```python
from build123d import *

# Parameters (mm, degrees)
SKETCH1_W                                  = 90
SKETCH1_H                                  = 65
SKETCH1_R                                  = 1.1
BOSS_EXTRUDE1_DEPTH                        = 1.6
CELL_AND_THERMISTOR_CONNECTORS_OUTLINE_W   = 29.4
CELL_AND_THERMISTOR_CONNECTORS_OUTLINE_H   = 11.5
CELL_AND_THERMISTOR_CONNECTORS_OUTLINE_W_2 = 27.4
CELL_AND_THERMISTOR_CONNECTORS_OUTLINE_H_2 = 9.5
CELL_AND_THERMISTOR_CONNECTORS_OUTLINE_W_3 = 11.4
CELL_AND_THERMISTOR_CONNECTORS_OUTLINE_W_4 = 9.4
CELL_AND_THERMISTOR_CONNECTORS_DEPTH       = 9.25
SKETCH3_W                                  = 13.5
SKETCH3_H                                  = 19.5
BOSS_EXTRUDE2_DEPTH                        = 19.5
SKETCH4_R                                  = 6
BOSS_EXTRUDE3_DEPTH                        = 13.5
SKETCH5_W                                  = 4.83
SKETCH5_H                                  = 17.78
JTAG_HEADER_DEPTH                          = 15.2
SKETCH6_W                                  = 7.37
SKETCH6_H                                  = 12.65
AUX_CAN_HEADER_DEPTH                       = 9.91


# Read off the part's stored shape, not the designer's step: Cell and thermistor connectors
with BuildPart() as part:
    # Sketch1 → Boss-Extrude1 (new body)
    with BuildSketch(Plane(origin=(0, 0, 0), x_dir=(1, 0, 0), z_dir=(0, 1, 0))):
        with Locations((45, 32.5)):
            Rectangle(SKETCH1_W, SKETCH1_H)
        with Locations(Location((5, 5, 0), (0, 0, 270))):
            Circle(SKETCH1_R, mode=Mode.SUBTRACT)
        with Locations(Location((5, 60, 0), (0, 0, 270))):
            Circle(SKETCH1_R, mode=Mode.SUBTRACT)
        with Locations(Location((55, 60, 0), (0, 0, 270))):
            Circle(SKETCH1_R, mode=Mode.SUBTRACT)
    extrude(amount=BOSS_EXTRUDE1_DEPTH)

    # Cell and thermistor connectors outline → Cell and thermistor connectors (add)
    # profile 1 of 2: a face of its own
    with BuildSketch(Plane.XZ):
        with Locations((29.7, -57.25)):
            Rectangle(CELL_AND_THERMISTOR_CONNECTORS_OUTLINE_W, CELL_AND_THERMISTOR_CONNECTORS_OUTLINE_H)
        with Locations((29.7, -57.25)):
            Rectangle(CELL_AND_THERMISTOR_CONNECTORS_OUTLINE_W_2, CELL_AND_THERMISTOR_CONNECTORS_OUTLINE_H_2, mode=Mode.SUBTRACT)
    # profile 2 of 2: a face of its own
    with BuildSketch(Plane.XZ):
        with Locations((71.7, -57.25)):
            Rectangle(CELL_AND_THERMISTOR_CONNECTORS_OUTLINE_W_3, CELL_AND_THERMISTOR_CONNECTORS_OUTLINE_H)
        with Locations((71.7, -57.25)):
            Rectangle(CELL_AND_THERMISTOR_CONNECTORS_OUTLINE_W_4, CELL_AND_THERMISTOR_CONNECTORS_OUTLINE_H_2, mode=Mode.SUBTRACT)
    extrude(amount=CELL_AND_THERMISTOR_CONNECTORS_DEPTH)

    # Sketch3 → Boss-Extrude2 (add)
    with BuildSketch(Plane(origin=(0, 1.6, 0), x_dir=(1, 0, 0), z_dir=(0, 1, 0))):
        with Locations((83.25, 13.757121209)):
            Rectangle(SKETCH3_W, SKETCH3_H)
    extrude(amount=BOSS_EXTRUDE2_DEPTH)

    # Sketch4 → Boss-Extrude3 (add)
    with BuildSketch(Plane(origin=(90, 0, 0), x_dir=(0, 0, -1), z_dir=(1, 0, 0))):
        with Locations(Location((13.757121209, 11.35, 0), (0, 0, 180))):
            Circle(SKETCH4_R)
    extrude(amount=BOSS_EXTRUDE3_DEPTH)

    # Sketch5 → JTAG header (add)
    with BuildSketch(Plane(origin=(0, 1.6, 0), x_dir=(1, 0, 0), z_dir=(0, 1, 0))):
        with Locations((52.415, 13.89)):
            Rectangle(SKETCH5_W, SKETCH5_H)
    extrude(amount=JTAG_HEADER_DEPTH)

    # Sketch6 → Aux. CAN header (add)
    with BuildSketch(Plane(origin=(0, 1.6, 0), x_dir=(1, 0, 0), z_dir=(0, 1, 0))):
        with Locations((66.203516114, 12.216109448)):
            Rectangle(SKETCH6_W, SKETCH6_H)
    extrude(amount=AUX_CAN_HEADER_DEPTH)


solid = part.part
```
The model under review builds one solid part; all positions refer to its coordinate system, in mm. A direction names the side the tool comes from. Coordinates: 2 decimals unless noted, no trailing zeros. Write each loop counter-clockwise with the first axis right and the second up, starting at its lowest first coordinate (ties: lowest second). Pieces come first, ordered by that corner, then holes. Notation, with made-up numbers: (2, -18) -> (19, -18) arc R29 cw to (19, 21) -> close; hole circle Ø1 at (-39, 12.5). An arc over 180 degrees is marked (long way). One line per item, written item: value. Start each with the question number.
Q1. Add section C-C, the plane z = -60. Give the boundary of the cut face in (x, y).
Q2. Clearance check with flat-ended pins moving along their axes: P1, Ø11, axis at x = 85.5, y = 15.5, coming from the -Z side; P2, Ø1.5, axis at x = 37, z = -50, coming from the +Y side; P3, Ø3, axis at x = 55, z = -60, coming from the -Y side; P4, Ø5, axis at y = -4.5, z = -12.5, coming from the +X side. State where each tip first meets the part, or that it passes through.
Q3. Add section B-B, the plane x = 5. Give the boundary of the cut face in (y, z), then the cut area to 3 significant figures.
Q4. Add section A-A, the plane y = -4. Give the boundary of the cut face in (x, z), then the cut area to 3 significant figures.
Q5. The part is to be moulded in two halves that separate along Z. For faces 1 (the face through (30, 0, -57)), 2 (the face through (66, 6, -5.891)), 3 (the face through (72, -5, -52.5)), 4 (the face through (54.83, 9, -14)), say which applies: +Z half, -Z half, draft (parallel to the pull), parting line (faces both ways), or undercut.
Q6. Add section D-D, the plane y = 8. Give the boundary of the cut face in (x, z).
Q7. For faces 5 (the face through (67, -5, -57)), 6 (the face through (66, 11.51, -12)), 7 (the face through (50, 9, -14)), list the 3-axis set-ups (+Z, -Z, +X, -X, +Y, -Y) from which the entire face can be reached by the end or side of a thin tool; tool diameter is ignored.
Q8. To check wall thickness, follow probe 1 along X at (y, z) = (0.4, -60); probe 2 along X at (y, z) = (8, -15); probe 3 along X at (y, z) = (14.5, -6). State the ranges of each line that lie inside material, in increasing order.
Response:
1. outline: (0, 0) -> (3.9, 0) -> (3.9, 1.6) -> (0, 1.6) -> close; (6.1, 0) -> (15, 0) -> (15, -9.25) -> (16, -9.25) -> (16, 0) -> (43.4, 0) -> (43.4, -9.25) -> (44.4, -9.25) -> (44.4, 0) -> (53.9, 0) -> (53.9, 1.6) -> (6.1, 1.6) -> close; (56.1, 0) -> (66, 0) -> (66, -9.25) -> (67, -9.25) -> (67, 0) -> (76.4, 0) -> (76.4, -9.25) -> (77.4, -9.25) -> (77.4, 0) -> (90, 0) -> (90, 1.6) -> (56.1, 1.6) -> close
2. P1: z = -23.51
2. P2: y = 1.6
2. P3: y = 0
2. P4: through
3. outline: (0, -65) -> (1.6, -65) -> (1.6, -61.1) -> (0, -61.1) -> close; (0, -58.9) -> (1.6, -58.9) -> (1.6, -6.1) -> (0, -6.1) -> close; (0, -3.9) -> (1.6, -3.9) -> (1.6, 0) -> (0, 0) -> close
3. area: 97.0 mm²
4. outline: (15, -63) -> (44.4, -63) -> (44.4, -51.5) -> (15, -51.5) -> close; (66, -63) -> (77.4, -63) -> (77.4, -51.5) -> (66, -51.5) -> close; hole (16, -62) -> (43.4, -62) -> (43.4, -52.5) -> (16, -52.5) -> close; hole (67, -62) -> (76.4, -62) -> (76.4, -52.5) -> (67, -52.5) -> close
4. area: 120 mm²
5. face 1: undercut
5. face 2: +Z half
5. face 3: undercut
5. face 4: draft
6. outline: (50, -22.78) -> (54.83, -22.78) -> (54.83, -5) -> (50, -5) -> close; (62.52, -18.54) -> (69.89, -18.54) -> (69.89, -5.89) -> (62.52, -5.89) -> close; (76.5, -23.51) -> (90, -23.51) -> (90, -18.73) -> (103.5, -18.73) -> (103.5, -8.78) -> (90, -8.78) -> (90, -4.01) -> (76.5, -4.01) -> close
7. face 5: -Y
7. face 6: +Z, -Z, +Y
7. face 7: +Z, -Z, -X, +Y
8. probe 1: 0 to 3.9, 6.1 to 53.9, 56.1 to 90
8. probe 2: 50 to 54.83, 62.52 to 69.89, 76.5 to 103.5
8. probe 3: 50 to 54.83, 76.5 to 90
